from build123d import *

# Parameters (mm, degrees)
SKETCH18_W                 = 25.4
SKETCH18_H                 = 25.4
BOSS_EXTRUDE3_DEPTH        = 50.8
F_1_2_0_5_DIAMETER_HOLE2_D = 12.7
SKETCH26_R                 = 3.175
CUT_EXTRUDE10_DEPTH        = 12.7
SKETCH27_R                 = 7.9375
CUT_EXTRUDE11_DEPTH        = 3.175
CUT_EXTRUDE12_START        = -12.7
SKETCH28_R                 = 3.175
CUT_EXTRUDE12_DEPTH        = 12.7
CUT_EXTRUDE13_START        = -3.175
SKETCH29_R                 = 7.9375
CUT_EXTRUDE13_DEPTH        = 3.175


with BuildPart() as part:
    # Sketch18 → Boss-Extrude3 (new, symmetric)
    with BuildSketch(Plane.XY):
        Rectangle(SKETCH18_W, SKETCH18_H)
    extrude(amount=BOSS_EXTRUDE3_DEPTH, both=True)

    # 1/2 (0.5) Diameter Hole2 (through all)
    with Locations(Plane.XY.offset(50.8)):
        with Locations((0, 0)):
            Hole(F_1_2_0_5_DIAMETER_HOLE2_D / 2)

    # Sketch26 → Cut-Extrude10 (cut)
    with BuildSketch(Plane(origin=(0, 12.7, 0), x_dir=(1, 0, 0), z_dir=(0, 1, 0))):
        with Locations(Location((0, -38.1, 0), (0, 0, 180))):
            Circle(SKETCH26_R)
        with Locations(Location((0, -3.175, 0), (0, 0, 180))):
            Circle(SKETCH26_R)
        with Locations(Location((0, 38.1, 0), (0, 0, 180))):
            Circle(SKETCH26_R)
    extrude(amount=-CUT_EXTRUDE10_DEPTH, mode=Mode.SUBTRACT)

    # Sketch27 → Cut-Extrude11 (cut)
    with BuildSketch(Plane(origin=(0, 12.7, 0), x_dir=(1, 0, 0), z_dir=(0, 1, 0))):
        with Locations(Location((0, 38.1, 0), (0, 0, 180))):
            Circle(SKETCH27_R)
        with Locations(Location((0, -3.175, 0), (0, 0, 180))):
            Circle(SKETCH27_R)
        with Locations(Location((0, -38.1, 0), (0, 0, 180))):
            Circle(SKETCH27_R)
    extrude(amount=-CUT_EXTRUDE11_DEPTH, mode=Mode.SUBTRACT)

    # Sketch28 → Cut-Extrude12 (cut)
    with BuildSketch(Plane.XZ.offset(12.7).offset(CUT_EXTRUDE12_START)):
        with Locations(Location((0, 3.175, 0), (0, 0, 180))):
            Circle(SKETCH28_R)
    extrude(amount=CUT_EXTRUDE12_DEPTH, mode=Mode.SUBTRACT)

    # Sketch29 → Cut-Extrude13 (cut)
    with BuildSketch(Plane(origin=(0, -12.7, 0), x_dir=(-1, 0, 0), z_dir=(0, -1, 0)).offset(CUT_EXTRUDE13_START)):
        with Locations((0, -3.175)):
            Circle(SKETCH29_R)
    extrude(amount=CUT_EXTRUDE13_DEPTH, mode=Mode.SUBTRACT)


solid = part.part
Source: CAD feature listing. Evaluate the final solid. Frame: model axes, mm. A direction names the side the tool comes from. Give positions to 0.01 mm unless a question says otherwise; leave off trailing zeros. Write each loop counter-clockwise with the first axis right and the second up, starting at its lowest first coordinate (ties: lowest second). Pieces come first, ordered by that corner, then holes. Notation, with made-up numbers: (-17, 54) - (-7, 54) arc R13 ccw to (-7, 70) - close; hole circle Ø5 at (9, -7). An arc over 180 degrees is marked (long way). Write item = value, one per line. Start each with the question number.
Q1. Material intervals for probe 1 along Z at (x, y) = (0, 7.6) (3 decimals); probe 2 along Z at (x, y) = (0, 10.75); probe 3 along Z at (x, y) = (0, -8.3), sorted ascending.
Q2. Pin query (flat end, axial travel): pin 1 Ø5.5 at (x, z) = (0, 3.175) entering from +Y; pin 2 Ø8.5 at (x, z) = (0, -38.1) entering from +Y (3 decimals); pin 3 Ø8.5 at (x, z) = (0, 3.175) entering from -Y (3 decimals). Return the tip coordinate at first contact, or that it passes through.
Q3. Cut plane B-B, the plane y = 0. Return loops of the section in (x, z).
Q4. Cut plane A-A, the plane z = 22.5. Return loops of the section in (x, y), then the cut area to 3 significant figures.
Q5. Reachability of faces 4 (the flat face through (-3.4, -9.525, 3.1)), 5 (the cylindrical face through (1.721, 11.135, -4.574)), 6 (the flat face through (-3, 6, 50.8)) from +Z, -Z, +X, -X, +Y, -Y: full face, straight path, thin tool, end or side. Return the list, or none.
Q6. Cut plane C-C, the plane x = 4.5. Return loops of the section in (y, z) (3 decimals).
Q7. Draft query along Z for faces 1 (the flat face through (-3, 6, -50.8)), 2 (the flat face through (-3.4, 9.525, -38)), 3 (the flat face through (12.7, 0, 1)). Return one class per face: +Z half, -Z half, draft (parallel to the pull), parting line (faces both ways), or undercut.
Computed values:
q1.probe_1 = -50.8 to -41.275, -34.925 to 0, 6.35 to 34.925, 41.275 to 50.8
q1.probe_2 = -50.8 to -46.04, -30.16 to -4.76, 11.11 to 30.16, 46.04 to 50.8
q1.probe_3 = -50.8 to 0, 6.35 to 50.8
q2.pin_1 = through
q2.pin_2 = 9.525
q2.pin_3 = -9.525
q3.outline = (-12.7, -50.8) - (-6.35, -50.8) - (-6.35, 50.8) - (-12.7, 50.8) - close; (6.35, -50.8) - (12.7, -50.8) - (12.7, 50.8) - (6.35, 50.8) - close
q4.outline = (-12.7, -12.7) - (12.7, -12.7) - (12.7, 12.7) - (-12.7, 12.7) - close; hole circle Ø12.7 at (0, 0)
q4.area = 518 mm²
q5.face_4 = -Y
q5.face_5 = +Y
q5.face_6 = +Z, +X, -X, +Y, -Y
q6.outline = (-12.7, -50.8) - (-4.48, -50.8) - (-4.48, 50.8) - (-12.7, 50.8) - (-12.7, 9.714) - (-9.525, 9.714) - (-9.525, -3.364) - (-12.7, -3.364) - close; (4.48, -50.8) - (12.7, -50.8) - (12.7, -44.639) - (9.525, -44.639) - (9.525, -31.561) - (12.7, -31.561) - (12.7, -3.364) - (9.525, -3.364) - (9.525, 9.714) - (12.7, 9.714) - (12.7, 31.561) - (9.525, 31.561) - (9.525, 44.639) - (12.7, 44.639) - (12.7, 50.8) - (4.48, 50.8) - close
q7.face_1 = -Z half
q7.face_2 = undercut
q7.face_3 = draft
